from build123d import *

# Parameters (mm, degrees)
BOSS_EXTRUDE1_DEPTH = 12.7
FILLET1_R           = 7.62
FILLET3_R           = 1.27
SHELL1_T            = -1.778


with BuildPart() as part:
    # Sketch2 → Boss-Extrude1 (new body)
    with BuildSketch(Plane(origin=(0, 0, 0), x_dir=(1, 0, 0), z_dir=(0, 1, 0))):
        with BuildLine():
            Line((-50.8, -58.42), (50.8, -58.42))
            ThreePointArc((50.8, -58.42), (56.188153673, -56.188153673), (58.42, -50.8))
            Line((58.42, -50.8), (58.42, 50.8))
            ThreePointArc((58.42, 50.8), (56.188153673, 56.188153673), (50.8, 58.42))
            Line((50.8, 58.42), (-50.8, 58.42))
            ThreePointArc((-50.8, 58.42), (-56.188153673, 56.188153673), (-58.42, 50.8))
            Line((-58.42, 50.8), (-58.42, -50.8))
            ThreePointArc((-58.42, -50.8), (-56.188153673, -56.188153673), (-50.8, -58.42))
        make_face()
    extrude(amount=BOSS_EXTRUDE1_DEPTH)

    # Fillet1
    # the kernel refuses this fillet: 7.62 mm, written as the material it takes off along each edge
    with BuildSketch(Plane(origin=(58.42, 12.7, 69.85), x_dir=(0, -1, 0), z_dir=(0, 0, -1)), Plane(origin=(-58.42, 12.7, -69.85), x_dir=(0, -1, 0), z_dir=(0, 0, 1))) as fillet1_piece_1:
        with BuildLine():
            CenterArc((FILLET1_R, FILLET1_R), FILLET1_R, 180, 90)
            Line((0, FILLET1_R), (0, 0))
            Line((0, 0), (FILLET1_R, 0))
        make_face()
    extrude(amount=139.7, mode=Mode.SUBTRACT)

    # Fillet3
    # the kernel refuses this fillet: 1.27 mm, written as the material it takes off along each edge
    with BuildSketch(Plane(origin=(53.975, 12.7, -58.42), x_dir=(0, 0, 1), z_dir=(-1, 0, 0))) as fillet3_piece_1:
        with BuildLine():
            CenterArc((FILLET3_R, -FILLET3_R), FILLET3_R, 90, 90)
            Line((0, -FILLET3_R), (0, 0))
            Line((0, 0), (FILLET3_R, 0))
        make_face()
    extrude(amount=107.95, mode=Mode.SUBTRACT)
    with BuildSketch(Plane(origin=(-53.975, 12.7, 58.42), x_dir=(0, -1, 0), z_dir=(1, 0, 0))) as fillet3_piece_2:
        with BuildLine():
            CenterArc((FILLET3_R, FILLET3_R), FILLET3_R, 180, 90)
            Line((0, FILLET3_R), (0, 0))
            Line((0, 0), (FILLET3_R, 0))
        make_face()
    extrude(amount=107.95, mode=Mode.SUBTRACT)

    # Shell1
    shell1_openings = [part.faces().sort_by_distance(p)[0] for p in [
        (0, 0, 0),
    ]]
    offset(amount=SHELL1_T, openings=shell1_openings)


solid = part.part
Read the model definition and answer for the solid it produces. Units are mm, in the model's axes. A direction names the side the tool comes from. Coordinates: 2 decimals unless noted, no trailing zeros. Write each loop counter-clockwise with the first axis right and the second up, starting at its lowest first coordinate (ties: lowest second). Pieces come first, ordered by that corner, then holes. Notation, with made-up numbers: (81.25, 51) - (96.25, 51) arc R18 ccw to (96.25, 86) - close; hole circle Ø4 at (2, 64.25). An arc over 180 degrees is marked (long way). One line per question, with ' | ' between items.
Q1. Find section C-C, the plane z = 5. Write down the section's boundary in (x, y).
Result set:
outline: (-58.42, 0) - (-56.64, 0) - (-56.64, 5.08) arc R5.84 cw to (-50.8, 10.92) - (50.8, 10.92) arc R5.84 cw to (56.64, 5.08) - (56.64, 0) - (58.42, 0) - (58.42, 5.08) arc R7.62 ccw to (50.8, 12.7) - (-50.8, 12.7) arc R7.62 ccw to (-58.42, 5.08) - close
Q2. Find section B-B, the plane x = -32. Write down the section's boundary in (y, z), plus the area to 3 significant figures.
Result set:
outline: (0, -58.42) - (11.43, -58.42) arc R1.27 ccw to (12.7, -57.15) - (12.7, 57.15) arc R1.27 ccw to (11.43, 58.42) - (0, 58.42) - (0, 56.64) - (10.92, 56.64) - (10.92, -56.64) - (0, -56.64) - close | area: 246 mm^2
Q3. Find section A-A, the plane y = 3.25. Write down the section's boundary in (x, z).
Result set:
outline: (-58.42, -50.8) arc R7.62 ccw to (-50.8, -58.42) - (50.8, -58.42) arc R7.62 ccw to (58.42, -50.8) - (58.42, 50.8) arc R7.62 ccw to (50.8, 58.42) - (-50.8, 58.42) arc R7.62 ccw to (-58.42, 50.8) - close; hole (-56.64, -50.8) arc R5.84 ccw to (-50.8, -56.64) - (50.8, -56.64) arc R5.84 ccw to (56.64, -50.8) - (56.64, 50.8) arc R5.84 ccw to (50.8, 56.64) - (-50.8, 56.64) arc R5.84 ccw to (-56.64, 50.8) - close
Q4. For faces 5 (the flat face through (-1, 12.7, -1)), 6 (the cylindrical face through (54.2, 4.17, -55.55)), determine the directions among +Z, -Z, +X, -X, +Y, -Y from which every point of the face is accessible in a straight line to the end or side of a thin tool.
Result set:
face 5: +Z, -Z, +X, -X, +Y | face 6: -Y
Q5. Each of these flat-tipped pins is pushed along its axis until it touches: P1, Ø1.5, axis at x = -20.5, z = 3.5, coming from the -Y side; P2, Ø4, axis at y = 10.5, z = -44.5, coming from the +X side; P3, Ø6, axis at y = 8, z = -5, coming from the -X side. Where does it stop, or does it pass through?
Result set:
P1: y = 10.92 | P2: x = 57.61 | P3: x = -58.42
Q6. Consider L1, parallel to X at y = 3.5, z = 5.5; L2, parallel to Y at x = 40.5, z = -25. Determine where each line is inside the solid, lowest interval first. Write a range as [from, to].
Result set:
L1: [-58.42, -56.64], [56.64, 58.42] | L2: [10.92, 12.7]
Q7. Determine the mould class of faces 1 (the cylindrical face through (-54.885, 4.171, -54.976)), 2 (the cylindrical face through (-56.129, 10.527, -0.813)), 3 (the cylindrical face through (55.1, 4.71, 57.09)), 4 (the cylindrical face through (54.885, 9.256, 0.793)) for opening direction X: +X half, -X half, draft (parallel to the pull), parting line (faces both ways), or undercut.
Result set:
face 1: undercut | face 2: -X half | face 3: +X half | face 4: undercut
